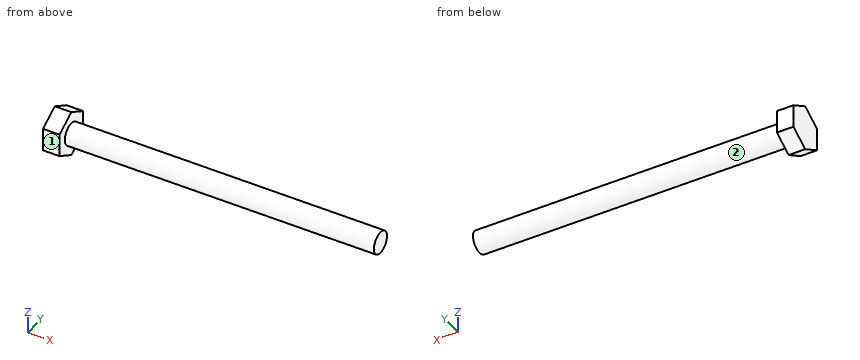
Autodesk Inventor part; units mm, degrees
ref_plane "YZ Plane" through (0, 0, 0) normal (1, 0, 0) x (0, 1, 0)
ref_plane "XZ Plane" through (0, 0, 0) normal (0, 1, 0) x (-1, 0, 0)
ref_plane "XY Plane" through (0, 0, 0) normal (0, 0, 1) x (1, 0, 0)
sketch "Náčrt1" plane through (0, 0, 0) normal (1, 0, 0) x (0, 1, 0)
  line L0 (0, -10.3923) -> (-9, -5.1962)
  line L1 (-9, -5.1962) -> (-9, 5.1962)
  line L2 (-9, 5.1962) -> (0, 10.3923)
  line L3 (0, 10.3923) -> (9, 5.1962)
  line L4 (9, 5.1962) -> (9, -5.1962)
  line L5 (9, -5.1962) -> (0, -10.3923)
  point P0 (0, 0)
  point P1 (0, 0)
  dimension "d0" = 18
extrude "Vysunutí1" add sketch "Náčrt1" along normal blind 7.5
sketch "Náčrt2" plane through (7.5, 0, 0) normal (1, 0, 0) x (0, 0, -1)
  circle A0 centre (0, 0) radius 5
  dimension "d3" = 10
extrude "Vysunutí2" add sketch "Náčrt2" along normal blind 140
thread "Závit1"
properties part number "Šrouv M12x160"
Input: part model. Units: mm. Frame: model coordinates. Face numbers are marked on the shaded views. A direction names the side the tool comes from. Coordinates: 2 decimals unless noted, no trailing zeros. Write each loop counter-clockwise with the first axis right and the second up, starting at its lowest first coordinate (ties: lowest second). Pieces come first, ordered by that corner, then holes. Notation, with made-up numbers: M 34.5,-19 L 91.5,-19 A35 ccw 91.5,13 Z; hole C -22.75,63.5 d6. An arc over 180 degrees is marked long. Answer as a JSON object with one key per item and string values. Group by question number.
(1) Section D-D on z = -7.25. Output: boundary loops of the cut face in (x, y), plus the area to 3 significant figures.
(2) Set-up query: the marked faces 1 and 2. Return all of +Z, -Z, +X, -X, +Y, -Y with unobstructed straight access to the full face (end or side cutting, diameter ignored); none if empty.
(3) Contact query for flat-ended pins moving along their axis: P1, Ø12, axis at x = 37, z = -7.5, coming from the +Y side; P2, Ø8, axis at x = 86.5, y = -0.5, coming from the -Z side; P3, Ø3, axis at x = 61, z = -5.5, coming from the +Y side. Output: stop coordinate, or through.
(4) Section C-C on x = 72.5. Output: boundary loops of the cut face in (y, z), plus the area to 3 significant figures.
(5) Section B-B on y = 3.5. Output: boundary loops of the cut face in (x, z).
(6) Section A-A on z = 0. Output: boundary loops of the cut face in (x, y).
(7) Ray query, line 1 along X through (y, z) = (-7.5, -2.75); line 2 along Z through (x, y) = (47.5, -0.25); line 3 along Z through (x, y) = (90.5, -1.25). Return the intervals inside material, ascending. Write a range as [from, to].
Result set:
{
 "1": {"outline": "M 0,-5.44 L 7.5,-5.44 L 7.5,5.44 L 0,5.44 Z", "area": "81.6 mm2"},
 "2": {"face 1": "+Z, -Z, +X, -X, -Y", "face 2": "+X"},
 "3": {"P1": "stops at y = 4.77", "P2": "stops at z = -5", "P3": "stops at y = 3"},
 "4": {"outline": "C 0,0 d10", "area": "78.5 mm2"},
 "5": {"outline": "M 0,-8.37 L 7.5,-8.37 L 7.5,-3.57 L 147.5,-3.57 L 147.5,3.57 L 7.5,3.57 L 7.5,8.37 L 0,8.37 Z"},
 "6": {"outline": "M 0,-9 L 7.5,-9 L 7.5,-5 L 147.5,-5 L 147.5,5 L 7.5,5 L 7.5,9 L 0,9 Z"},
 "7": {"line 1": "x = [0, 7.5]", "line 2": "z = [-4.99, 4.99]", "line 3": "z = [-4.84, 4.84]"}
}
